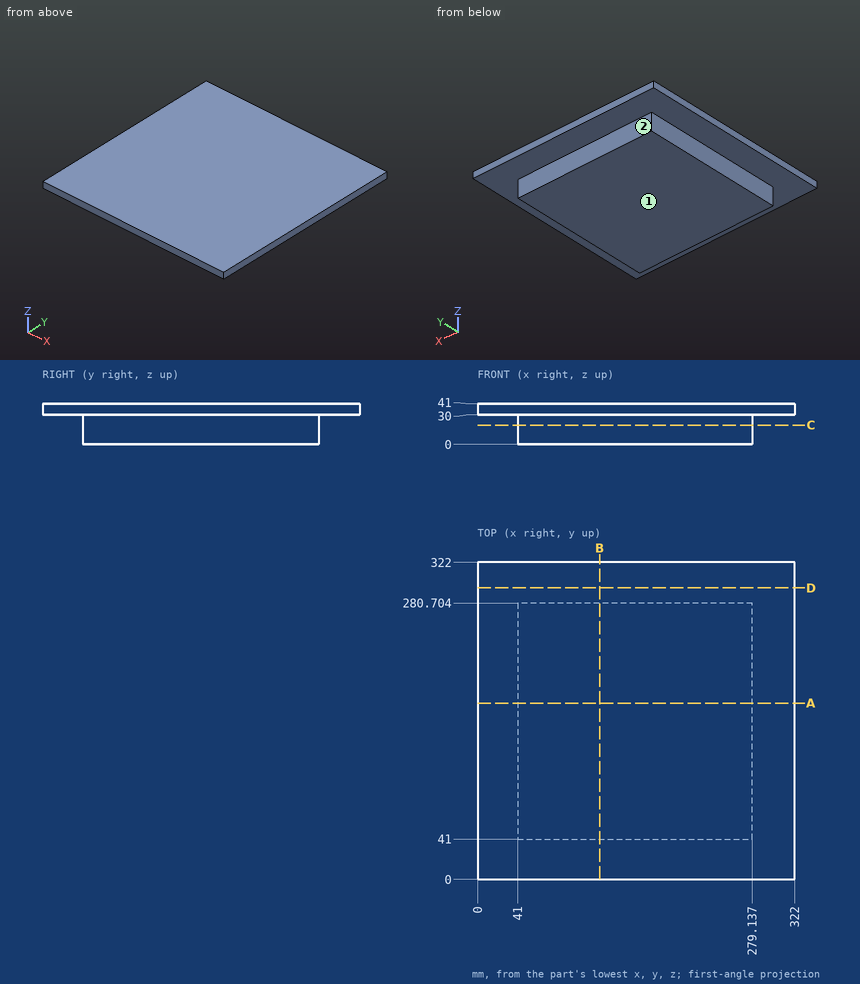
Check sheet for the drawn part. Datum: minimum x, y, z corner. Units: mm. A direction names the side the tool comes from. Round coordinates to 2 decimals unless told otherwise and drop trailing zeros. Order: outer loops, then holes, each group sorted by start corner. A loop starts at its lowest first (then second) coordinate and runs counter-clockwise, first axis right, second up.
1. Go/stop test with flat-tipped pins: P1, Ø9, axis at y = 124, z = 21.5, coming from the +X side; P2, Ø5, axis at x = 58.5, z = 26, coming from the -Y side; P3, Ø5, axis at x = 38, z = 5, coming from the +Y side; P4, Ø15, axis at y = 160.5, z = 10.5, coming from the -X side. Record where each tip stops, or that it passes through.
Final values:
P1: stops at x = 279.14
P2: stops at y = 41
P3: passes through
P4: stops at x = 41
2. Thickness scan on L1, parallel to X at y = 141, z = 9; L2, parallel to Y at x = 60, z = 12; L3, parallel to Z at x = 182, y = 29. Record the ranges inside material, lowest first.
Final values:
L1: x = 41 to 279.14
L2: y = 41 to 280.7
L3: z = 30 to 41
3. Section check B-B on x = 124. Record the cut outline in (y, z), then the cut area to 3 significant figures.
Final values:
outline: (0, 30) - (41, 30) - (41, 0) - (280.7, 0) - (280.7, 30) - (322, 30) - (322, 41) - (0, 41) - close
area: 10,700 mm2
4. Section check A-A on y = 179. Record the cut outline in (x, z).
Final values:
outline: (0, 30) - (41, 30) - (41, 0) - (279.14, 0) - (279.14, 30) - (322, 30) - (322, 41) - (0, 41) - close
5. Access from +Z, -Z, +X, -X, +Y, -Y to the whole of each face (thin tool, end or side, straight path). Record for the marked faces 1 and 2.
Final values:
face 1: -Z, +X, -X, +Y, -Y
face 2: -Z, +X, -X, +Y
6. Section check C-C on z = 19.5. Record the cut outline in (x, y).
Final values:
outline: (41, 41) - (279.14, 41) - (279.14, 280.7) - (41, 280.7) - close
7. Section check D-D on y = 296. Record the cut outline in (x, z), then the cut area to 3 significant figures.
Final values:
outline: (0, 30) - (322, 30) - (322, 41) - (0, 41) - close
area: 3,540 mm2
